from build123d import *

# Parameters (mm, degrees)
SKETCH1_R                = 30
SKETCH1_R_2              = 5
BOSS_EXTRUDE3_DEPTH      = 30
SKETCH2_R                = 19.858143103
CUT_EXTRUDE1_DEPTH       = 10
SKETCH3_R                = 2.771368275
CUT_EXTRUDE2_DEPTH       = 21
SKETCH4_R                = 6.5
SKETCH4_R_2              = 5
BOSS_EXTRUDE4_DEPTH      = 2
BOSS_EXTRUDE4_DEPTH_BACK = 7


with BuildPart() as part:
    # Sketch1 → Boss-Extrude3 (new body)
    with BuildSketch(Plane.XY):
        Circle(SKETCH1_R)
        Circle(SKETCH1_R_2, mode=Mode.SUBTRACT)
    extrude(amount=BOSS_EXTRUDE3_DEPTH)

    # Sketch2 → Cut-Extrude1 (cut)
    with BuildSketch(Plane.XY.offset(30)):
        Circle(SKETCH2_R)
    cut_extrude1 = extrude(amount=-CUT_EXTRUDE1_DEPTH, mode=Mode.SUBTRACT)

    # Mirror1: Cut-Extrude1 across plane
    add(cut_extrude1.mirror(Plane.XY), mode=Mode.SUBTRACT)

    # Sketch3 → Cut-Extrude2 (cut, through all)
    with BuildSketch(Plane.XY.offset(20)):
        with Locations((0, 12)):
            Circle(SKETCH3_R)
        with Locations((11.412678196, 3.708203932)):
            Circle(SKETCH3_R)
        with Locations((7.053423028, -9.708203932)):
            Circle(SKETCH3_R)
        with Locations((-7.053423028, -9.708203932)):
            Circle(SKETCH3_R)
        with Locations((-11.412678196, 3.708203932)):
            Circle(SKETCH3_R)
    extrude(amount=-CUT_EXTRUDE2_DEPTH, mode=Mode.SUBTRACT)

    # Sketch4 → Boss-Extrude4 (add, two sides)
    with BuildSketch(Plane.XY.offset(20)) as boss_extrude4_sk:
        Circle(SKETCH4_R)
        Circle(SKETCH4_R_2, mode=Mode.SUBTRACT)
    extrude(amount=BOSS_EXTRUDE4_DEPTH)
    extrude(boss_extrude4_sk.sketch, amount=-BOSS_EXTRUDE4_DEPTH_BACK)

    # Sketch5 → Cut-Revolve1 (revolve, cut)
    with BuildSketch(Plane(origin=(0, 0, 0), x_dir=(1, 0, 0), z_dir=(0, 1, 0))):
        Polygon((30, -3), (22.205771366, -7.5), (22.205771366, -22.5), (30, -27), align=None)
    revolve(axis=Axis((0, 0, 0), (0, 0, -1)), mode=Mode.SUBTRACT)


solid = part.part
Design review of the part built by this model. Coordinates are the model's own, in mm. A direction names the side the tool comes from. Coordinates: 2 decimals unless noted, no trailing zeros. Order: outer loops, then holes, each group sorted by start corner. A loop starts at its lowest first (then second) coordinate and runs counter-clockwise, first axis right, second up. Notation, with made-up numbers: M 9.25,41 L 19.25,41 A32 cw 19.25,72 Z; hole C 27.25,-24.75 d7. An arc over 180 degrees is marked long. Use a Markdown table: item, result.
(1) Add section B-B (x = 0). Give the boundary of the cut face in (y, z).
Worked answers:
| item | result |
|---|---|
| outline | M -30,0 L -5,0 L -5,22 L -6.5,22 L -6.5,20 L -19.86,20 L -19.86,30 L -30,30 L -30,27 L -22.21,22.5 L -22.21,7.5 L -30,3 Z; M 5,0 L 9.23,0 L 9.23,20 L 6.5,20 L 6.5,22 L 5,22 Z; M 14.77,0 L 30,0 L 30,3 L 22.21,7.5 L 22.21,22.5 L 30,27 L 30,30 L 19.86,30 L 19.86,20 L 14.77,20 Z |
(2) Wall thickness on probe 1 along Y at (x, z) = (0, 11); probe 2 along Y at (x, z) = (0, 27.75); probe 3 along X at (y, z) = (-7.5, 17.25): over which ranges is each line inside the solid? List them lowest first.
Worked answers:
| item | result |
|---|---|
| probe 1 | y = -22.21 to -5, 5 to 9.23, 14.77 to 22.21 |
| probe 2 | y = -30 to -19.86, 19.86 to 30 |
| probe 3 | x = -20.9 to -8.73, -5.38 to 5.38, 8.73 to 20.9 |
(3) Draft analysis for pull direction Z (two halves, no side actions). For faces 1 (the conical face through (21.5, -6.8, 7.3)), 2 (the conical face through (21.645, -6.816, 22.782)), 3 (the cylindrical face through (8.644, 3.83, 10.14)), 4 (the flat face through (2, -5, 22)), state which applies: released by +Z, released by -Z, zero draft, split by the parting line, or undercut.
Worked answers:
| item | result |
|---|---|
| face 1 | undercut |
| face 2 | undercut |
| face 3 | zero draft |
| face 4 | released by +Z |
(4) Add section A-A (y = 0). Give the boundary of the cut face in (x, z).
Worked answers:
| item | result |
|---|---|
| outline | M -30,0 L -5,0 L -5,22 L -6.5,22 L -6.5,20 L -19.86,20 L -19.86,30 L -30,30 L -30,27 L -22.21,22.5 L -22.21,7.5 L -30,3 Z; M 5,0 L 30,0 L 30,3 L 22.21,7.5 L 22.21,22.5 L 30,27 L 30,30 L 19.86,30 L 19.86,20 L 6.5,20 L 6.5,22 L 5,22 Z |
(5) Add section D-D (z = 23.5). Give the boundary of the cut face in (x, y), then the cut area to 3 significant figures.
Worked answers:
| item | result |
|---|---|
| outline | C 0,0 d47.88; hole C 0,0 d39.72 |
| area | 561 mm2 |
(6) For P1, Ø8, axis at y = -6, z = 6.5, coming from the -X side; P2, Ø4.5, axis at x = 7.05, y = -9.71, coming from the +Z side; P3, Ø1, axis at x = -3, z = 14, coming from the -Y side; P4, Ø4, axis at x = -15, z = 8, coming from the -Y side, all flat-tipped, find the tip position at first contact; note any pin that passes through.
Worked answers:
| item | result |
|---|---|
| P1 | stops at x = -29.72 |
| P2 | passes through |
| P3 | stops at y = -22.06 |
| P4 | stops at y = -20 |
(7) For faces 5 (the flat face through (-5, 5, 20)), 6 (the cylindrical face through (-9.1, -7.84, 10.14)), 7 (the cylindrical face through (21.18, -6.67, 15.1)), list the 3-axis set-ups (+Z, -Z, +X, -X, +Y, -Y) from which the entire face can be reached by the end or side of a thin tool; tool diameter is ignored.
Worked answers:
| item | result |
|---|---|
| face 5 | +Z |
| face 6 | +Z, -Z |
| face 7 | none |
(8) Add section C-C (z = 15.75). Give the boundary of the cut face in (x, y).
Worked answers:
| item | result |
|---|---|
| outline | C 0,0 d44.41; hole C -11.41,3.71 d5.54; hole C -7.05,-9.71 d5.54; hole C 0,0 d10; hole C 0,12 d5.54; hole C 7.05,-9.71 d5.54; hole C 11.41,3.71 d5.54 |
